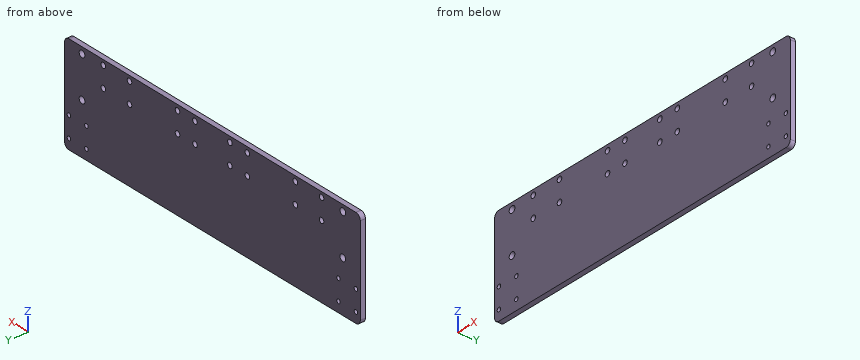
```python
from build123d import *

# Parameters (mm, degrees)
SKETCH_1_R          = 2.6
SKETCH_1_R_2        = 1.6
SKETCH_1_R_3        = 1.600000005
EXTRUDE_1_DEPTH     = 4
SKETCH_2_R          = 2.1
CUT_EXTRUDE_1_DEPTH = 10
SKETCH_3_R          = 2.1
CUT_EXTRUDE_2_DEPTH = 10


with BuildPart() as part:
    # 草图1 → 凸台-拉伸1 (new body)
    with BuildSketch(Plane(origin=(0, 0, 0), x_dir=(1, 0, 0), z_dir=(0, 1, 0))):
        with BuildLine():
            Line((43.366933006, 50.318582259), (43.366933006, 19.318582258))
            Line((43.366933006, 19.318582258), (43.366933006, -18.681417742))
            ThreePointArc((43.366933006, -18.681417742), (42.19536013, -21.509844867), (39.366933005, -22.681417742))
            Line((39.366933005, -22.681417742), (-223.633066993, -22.681417742))
            ThreePointArc((-223.633066993, -22.681417742), (-226.461494119, -21.509844867), (-227.633066994, -18.681417742))
            Line((-227.633066994, -18.681417742), (-227.633066994, 19.318582258))
            Line((-227.633066994, 19.318582258), (-227.633066994, 50.318582259))
            ThreePointArc((-227.633066994, 50.318582259), (-226.461494119, 53.147009385), (-223.633066993, 54.31858226))
            Line((-223.633066993, 54.31858226), (39.366933005, 54.31858226))
            ThreePointArc((39.366933005, 54.31858226), (42.19536013, 53.147009385), (43.366933006, 50.318582259))
        make_face()
        with Locations(Location((-211.63306699, 14.318582258, 0), (0, 0, 90))):
            Circle(SKETCH_1_R, mode=Mode.SUBTRACT)
        with Locations(Location((-211.63306699, -17.681417742, 0), (0, 0, 90))):
            Circle(SKETCH_1_R, mode=Mode.SUBTRACT)
        with Locations(Location((27.36693301, -17.681417742, 0), (0, 0, 270))):
            Circle(SKETCH_1_R, mode=Mode.SUBTRACT)
        with Locations(Location((-207.63306699, 30.318582258, 0), (0, 0, 270))):
            Circle(SKETCH_1_R_2, mode=Mode.SUBTRACT)
        with Locations(Location((-207.63306699, 46.31858226, 0), (0, 0, 90))):
            Circle(SKETCH_1_R_2, mode=Mode.SUBTRACT)
        with Locations(Location((-223.63306699, 30.318582258, 0), (0, 0, 270))):
            Circle(SKETCH_1_R_2, mode=Mode.SUBTRACT)
        with Locations(Location((-223.63306699, 46.31858226, 0), (0, 0, 90))):
            Circle(SKETCH_1_R_2, mode=Mode.SUBTRACT)
        with Locations(Location((27.36693301, 14.318582258, 0), (0, 0, 270))):
            Circle(SKETCH_1_R, mode=Mode.SUBTRACT)
        with Locations(Location((39.366933005, 30.318582258, 0), (0, 0, 90))):
            Circle(SKETCH_1_R_3, mode=Mode.SUBTRACT)
        with Locations(Location((23.36693301, 30.318582258, 0), (0, 0, 90))):
            Circle(SKETCH_1_R_2, mode=Mode.SUBTRACT)
        with Locations(Location((39.366933005, 46.31858226, 0), (0, 0, 270))):
            Circle(SKETCH_1_R_3, mode=Mode.SUBTRACT)
        with Locations(Location((23.36693301, 46.31858226, 0), (0, 0, 270))):
            Circle(SKETCH_1_R_2, mode=Mode.SUBTRACT)
    extrude(amount=EXTRUDE_1_DEPTH)

    # 草图2 → 切除-拉伸1 (cut)
    with BuildSketch(Plane(origin=(0, 4, 0), x_dir=(1, 0, 0), z_dir=(0, 1, 0))):
        with Locations(Location((-124.133066994, -2.381417742, 0), (0, 0, 90))):
            Circle(SKETCH_2_R)
        with Locations(Location((-124.133066994, -18.381417742, 0), (0, 0, 90))):
            Circle(SKETCH_2_R)
        with Locations(Location((-108.133066994, -18.381417742, 0), (0, 0, 90))):
            Circle(SKETCH_2_R)
        with Locations(Location((-108.133066994, -2.381417742, 0), (0, 0, 90))):
            Circle(SKETCH_2_R)
        with Locations(Location((-76.133066994, -2.381417742, 0), (0, 0, 270))):
            Circle(SKETCH_2_R)
        with Locations(Location((-76.133066994, -18.381417742, 0), (0, 0, 270))):
            Circle(SKETCH_2_R)
        with Locations(Location((-60.133066994, -18.381417742, 0), (0, 0, 270))):
            Circle(SKETCH_2_R)
        with Locations(Location((-60.133066994, -2.381417742, 0), (0, 0, 270))):
            Circle(SKETCH_2_R)
    extrude(amount=-CUT_EXTRUDE_1_DEPTH, mode=Mode.SUBTRACT)

    # 草图3 → 切除-拉伸2 (cut)
    with BuildSketch(Plane(origin=(0, 4, 0), x_dir=(1, 0, 0), z_dir=(0, 1, 0))):
        with Locations(Location((7.866933006, -18.681417742, 0), (0, 0, 270))):
            Circle(SKETCH_3_R)
        with Locations(Location((-16.133066994, -18.681417742, 0), (0, 0, 270))):
            Circle(SKETCH_3_R)
        with Locations(Location((7.866933006, -2.681417742, 0), (0, 0, 270))):
            Circle(SKETCH_3_R)
        with Locations(Location((-16.133066994, -2.681417742, 0), (0, 0, 270))):
            Circle(SKETCH_3_R)
        with Locations(Location((-168.133066994, -18.681417742, 0), (0, 0, 90))):
            Circle(SKETCH_3_R)
        with Locations(Location((-168.133066994, -2.681417742, 0), (0, 0, 90))):
            Circle(SKETCH_3_R)
        with Locations(Location((-192.133066994, -18.681417742, 0), (0, 0, 90))):
            Circle(SKETCH_3_R)
        with Locations(Location((-192.133066994, -2.681417742, 0), (0, 0, 90))):
            Circle(SKETCH_3_R)
    extrude(amount=-CUT_EXTRUDE_2_DEPTH, mode=Mode.SUBTRACT)


solid = part.part
```
The listing builds one solid part. Answer for the finished solid, in the listing's coordinates (mm). Coordinates: 2 decimals unless noted, no trailing zeros. Loops run counter-clockwise (first coordinate to the right, second up) from the corner with the lowest first, then second, coordinate; pieces in that order, holes last. Notation, with made-up numbers: (-31, -9) - (10, -9) arc R21 cw to (10, -4) - close; hole circle Ø1 at (3.5, 89). An arc over 180 degrees is marked (long way). Write item = value, one per line.
1) Section A-A (z = -14.5) is taken. Determine the outline of the cut face in (x, y), plus the area to 3 significant figures.
Responses:
outline = (-227.63, 0) - (-214.23, 0) - (-214.23, 4) - (-227.63, 4) - close; (-209.04, 0) - (24.77, 0) - (24.77, 4) - (-209.04, 4) - close; (29.96, 0) - (43.37, 0) - (43.37, 4) - (29.96, 4) - close
area = 1,040 mm^2
2) Find the intervals of material crossed by line 1 along X through (y, z) = (2.15, -13); line 2 along Z through (x, y) = (9.5, 1.35), in increasing order.
Responses:
line_1 = -227.63 to -213.87, -209.39 to 25.13, 29.61 to 43.37
line_2 = -54.32 to 1.36, 4 to 17.36, 20 to 22.68
3) Section B-B (y = 0.8) is taken. Count the separate pieces of the cut face and the enclosed holes in it, plus the area to 3 significant figures.
Responses:
separate_pieces = 1
enclosed_holes = 28
area = 20,500 mm^2
4) This flat-tipped pin is pushed along its axis until it touches: P1, Ø5.5, axis at x = -192.13, z = 18.68, coming from the +Y side. Where does it stop, or does it pass through?
Responses:
P1 = 4
